Could you check a few things on this model? Use its own coordinates, in mm. A direction names the side the tool comes from. Coordinates: 2 decimals unless noted, no trailing zeros. Order: outer loops, then holes, each group sorted by start corner. A loop starts at its lowest first (then second) coordinate and runs counter-clockwise, first axis right, second up. Notation, with made-up numbers: M -8,-27 L 45,-27 A22 ccw 45,0 Z; hole C 79.25,54.5 d8. An arc over 180 degrees is marked long. Write item = value, one per line. Start each with the question number.
from build123d import *

# Parameters (mm, degrees)
SKETCH_1_W          = 10
SKETCH_1_H          = 10
SKETCH_1_W_2        = 8
SKETCH_1_H_2        = 8
EXTRUDE_1_DEPTH     = 110
SKETCH_2_R          = 1.6
CUT_EXTRUDE_1_DEPTH = 111.566721937
SKETCH_3_R          = 1.6
CUT_EXTRUDE_2_DEPTH = 111.566721937


with BuildPart() as part:
    # ｽｹｯﾁ1 → ﾎﾞｽ - 押し出し1 (new body)
    with BuildSketch(Plane.XY):
        Rectangle(SKETCH_1_W, SKETCH_1_H)
        Rectangle(SKETCH_1_W_2, SKETCH_1_H_2, mode=Mode.SUBTRACT)
    extrude(amount=EXTRUDE_1_DEPTH)

    # ｽｹｯﾁ2 → ｶｯﾄ - 押し出し1 (cut, through all)
    with BuildSketch(Plane(origin=(0, 5, 0), x_dir=(1, 0, 0), z_dir=(0, 1, 0))):
        with Locations(Location((0, -55, 0), (0, 0, 270))):
            Circle(SKETCH_2_R)
    extrude(amount=-CUT_EXTRUDE_1_DEPTH, mode=Mode.SUBTRACT)

    # ｽｹｯﾁ3 → ｶｯﾄ - 押し出し2 (cut, through all)
    with BuildSketch(Plane(origin=(5, 0, 0), x_dir=(0, 0, -1), z_dir=(1, 0, 0))):
        with Locations((-65, 0)):
            Circle(SKETCH_3_R)
        with Locations((-45, 0)):
            Circle(SKETCH_3_R)
    extrude(amount=-CUT_EXTRUDE_2_DEPTH, mode=Mode.SUBTRACT)


solid = part.part
(1) Imagine slicing it at D-D on z = 55. List the corners of the cut face in (x, y) for me.
(2) Imagine slicing it at B-B on x = -3. List the corners of the cut face in (y, z) for me, plus the area to 3 significant figures.
(3) Imagine slicing it at C-C on y = 0. List the corners of the cut face in (x, z) for me, plus the area to 3 significant figures.
(4) Please list where these lines run through material, in increasing order: probe 1 along X at (y, z) = (-2.75, 6); probe 2 along X at (y, z) = (-4.6, 55). Write a range as from..to.
(5) For faces 4 (the flat face through (2, 5, 54)), 5 (the flat face through (-2, -4, 54)), which set-ups out of +Z, -Z, +X, -X, +Y, -Y let a thin tool reach every point of the face, with its end or its side?
(6) Thinking about a two-plate mould opening in Y: for faces 1 (the flat face through (-2, 4, 54)), 2 (the flat face through (2, -5, 54)), 3 (the flat face through (5, 0, 54)), which applies, released by +Y, released by -Y, zero draft, split by the parting line, or undercut?
(7) Imagine slicing it at A-A on z = 38. List the corners of the cut face in (x, y) for me.
Response:
q1.outline = M -5,-5 L -1.6,-5 L -1.6,-4 L -4,-4 L -4,4 L -1.6,4 L -1.6,5 L -5,5 Z; M 1.6,-5 L 5,-5 L 5,5 L 1.6,5 L 1.6,4 L 4,4 L 4,-4 L 1.6,-4 Z
q2.outline = M -5,0 L -4,0 L -4,110 L -5,110 Z; M 4,0 L 5,0 L 5,110 L 4,110 Z
q2.area = 220 mm2
q3.outline = M -5,0 L -4,0 L -4,43.4 L -5,43.4 Z; M -5,46.6 L -4,46.6 L -4,63.4 L -5,63.4 Z; M -5,66.6 L -4,66.6 L -4,110 L -5,110 Z; M 4,0 L 5,0 L 5,43.4 L 4,43.4 Z; M 4,46.6 L 5,46.6 L 5,63.4 L 4,63.4 Z; M 4,66.6 L 5,66.6 L 5,110 L 4,110 Z
q3.area = 207 mm2
q4.probe_1 = -5..-4, 4..5
q4.probe_2 = -5..-1.6, 1.6..5
q5.face_4 = +Z, -Z, +X, -X, +Y
q5.face_5 = +Z, -Z
q6.face_1 = undercut
q6.face_2 = released by -Y
q6.face_3 = zero draft
q7.outline = M -5,-5 L 5,-5 L 5,5 L -5,5 Z; hole M -4,-4 L 4,-4 L 4,4 L -4,4 Z
